from build123d import *

# Parameters (mm, degrees)
BOSS_EXTRUDE1_DEPTH   = 30
SKETCH2_R             = 3
CUT_EXTRUDE1_DEPTH    = 30
SKETCH3_R             = 9.5
CUT_EXTRUDE2_DEPTH    = 6
SKETCH4_R             = 9.5
CUT_EXTRUDE3_DEPTH    = 6
CUT_EXTRUDE4_REACH    = 26
SKETCH5_R             = 5
SKETCH6_W             = 110
SKETCH6_H             = 20
CUT_EXTRUDE5_DEPTH    = 12
SKETCH7_W             = 110
SKETCH7_H             = 20
CUT_EXTRUDE6_DEPTH    = 12
SKETCH8_W             = 12
SKETCH8_H             = 30
BOSS_EXTRUDE2_DEPTH   = 32
CUT_EXTRUDE7_DEPTH    = 35
BOSS_EXTRUDE3_DEPTH   = 50
SKETCH11_R            = 1.5
CUT_EXTRUDE8_DEPTH    = 10
SKETCH13_R            = 1.5
CUT_EXTRUDE9_DEPTH    = 10
SKETCH12_R            = 1.5
CUT_EXTRUDE10_DEPTH   = 10
BODY_MOVE_COPY1_ANGLE = 90


with BuildPart() as part:
    # Sketch1 → Boss-Extrude1 (new body)
    with BuildSketch(Plane(origin=(0, 0, 0), x_dir=(0, 0, -1), z_dir=(1, 0, 0))):
        with BuildLine():
            Line((0, 30), (135, 30))
            ThreePointArc((135, 30), (150, 15), (135, 0))
            Line((135, 0), (0, 0))
            ThreePointArc((0, 0), (-15, 15), (0, 30))
        make_face()
    extrude(amount=BOSS_EXTRUDE1_DEPTH)

    # Sketch2 → Cut-Extrude1 (cut)
    with BuildSketch(Plane(origin=(30, 0, 0), x_dir=(0, 0, -1), z_dir=(1, 0, 0))):
        with Locations((0, 15)):
            Circle(SKETCH2_R)
    extrude(amount=-CUT_EXTRUDE1_DEPTH, mode=Mode.SUBTRACT)

    # Sketch3 → Cut-Extrude2 (cut)
    with BuildSketch(Plane(origin=(30, 0, 0), x_dir=(0, 0, -1), z_dir=(1, 0, 0))):
        with Locations((135, 15)):
            Circle(SKETCH3_R)
    extrude(amount=-CUT_EXTRUDE2_DEPTH, mode=Mode.SUBTRACT)

    # Sketch4 → Cut-Extrude3 (cut)
    with BuildSketch(Plane.ZY):
        with Locations((-135, 15)):
            Circle(SKETCH4_R)
    extrude(amount=-CUT_EXTRUDE3_DEPTH, mode=Mode.SUBTRACT)

    # Sketch5 → Cut-Extrude4 (cut, up to next)
    with BuildSketch(Plane.ZY.offset(-6), mode=Mode.PRIVATE) as cut_extrude4_sk1:
        with Locations((-135, 15)):
            Circle(SKETCH5_R)
    cut_extrude4_tool1 = extrude(cut_extrude4_sk1.sketch, amount=-CUT_EXTRUDE4_REACH, mode=Mode.PRIVATE) & part.part
    add(cut_extrude4_tool1.solids().sort_by_distance((6, 15, -135))[0], mode=Mode.SUBTRACT)

    # Sketch6 → Cut-Extrude5 (cut)
    with BuildSketch(Plane(origin=(30, 0, 0), x_dir=(0, 0, -1), z_dir=(1, 0, 0))):
        with Locations((67.5, 15)):
            Rectangle(SKETCH6_W, SKETCH6_H)
    extrude(amount=-CUT_EXTRUDE5_DEPTH, mode=Mode.SUBTRACT)

    # Sketch7 → Cut-Extrude6 (cut)
    with BuildSketch(Plane.ZY):
        with Locations((-67.5, 15)):
            Rectangle(SKETCH7_W, SKETCH7_H)
    extrude(amount=-CUT_EXTRUDE6_DEPTH, mode=Mode.SUBTRACT)

    # Sketch8 → Boss-Extrude2 (add)
    with BuildSketch(Plane.ZY.offset(-12)):
        with Locations((-97, 15)):
            Rectangle(SKETCH8_W, SKETCH8_H)
        with Locations((-151, 15)):
            Rectangle(SKETCH8_W, SKETCH8_H)
    extrude(amount=BOSS_EXTRUDE2_DEPTH)

    # Sketch9 → Cut-Extrude7 (cut)
    with BuildSketch(Plane(origin=(12, 0, 0), x_dir=(0, 0, -1), z_dir=(1, 0, 0))):
        with BuildLine():
            Line((145, 30), (145, 26.180339887))
            ThreePointArc((145, 26.180339887), (150, 15), (145, 3.819660113))
            Line((145, 3.819660113), (145, 0))
            Line((145, 0), (157, 0))
            Line((157, 0), (157, 30))
            Line((157, 30), (145, 30))
        make_face()
    extrude(amount=-CUT_EXTRUDE7_DEPTH, mode=Mode.SUBTRACT)

    # Sketch10 → Boss-Extrude3 (add)
    with BuildSketch(Plane(origin=(30, 0, 0), x_dir=(0, 0, -1), z_dir=(1, 0, 0))):
        with BuildLine():
            Line((135, 30), (145, 30))
            ThreePointArc((145, 30), (160, 15), (145, 0))
            Line((145, 0), (135, 0))
            ThreePointArc((135, 0), (150, 15), (135, 30))
        make_face()
    extrude(amount=-BOSS_EXTRUDE3_DEPTH)

    # Sketch11 → Cut-Extrude8 (cut)
    with BuildSketch(Plane.ZY.offset(20)):
        with Locations((-149.85, 10.350189987)):
            Circle(SKETCH11_R)
    extrude(amount=-CUT_EXTRUDE8_DEPTH, mode=Mode.SUBTRACT)

    # Sketch13 → Cut-Extrude9 (cut)
    with BuildSketch(Plane.ZY.offset(20)):
        with Locations((-149.85, 20.350189987)):
            Circle(SKETCH13_R)
        with Locations((-99.35, 20.350189987)):
            Circle(SKETCH13_R)
    extrude(amount=-CUT_EXTRUDE9_DEPTH, mode=Mode.SUBTRACT)

    # Sketch12 → Cut-Extrude10 (cut)
    with BuildSketch(Plane.ZY.offset(20)):
        with Locations((-99.35, 10.350189987)):
            Circle(SKETCH12_R)
    extrude(amount=-CUT_EXTRUDE10_DEPTH, mode=Mode.SUBTRACT)


with BuildPart() as part_1:
    # Body-Move/Copy1: moved
    add(part.part.rotate(Axis((5, 0, -72.5), (0, -1, 0)), BODY_MOVE_COPY1_ANGLE))


with BuildPart() as part_2:
    # Body-Move/Copy2: moved
    add(part_1.part.moved(Location((67.5, -15, 47.5))))


solid = part_2.part
The model under review builds one solid part; all positions refer to its coordinate system, in mm. A direction names the side the tool comes from. Give positions to 0.01 mm unless a question says otherwise; leave off trailing zeros. Order: outer loops, then holes, each group sorted by start corner. A loop starts at its lowest first (then second) coordinate and runs counter-clockwise, first axis right, second up. Notation, with made-up numbers: (9, -36.5) -> (53, -36.5) arc R8 cw to (53, -21.5) -> close; hole circle Ø4 at (85, 20.25). An arc over 180 degrees is marked (long way). Write item = value, one per line. Start each with the question number.
(1) Take a section at A-A (z = -45). Write out the cut boundary in (x, y).
(2) For L1, parallel to Y at x = 135, z = -15.5; L2, parallel to X at y = 3.75, z = -22; L3, parallel to Y at x = 99.35, z = -43.5, list the stretches that pass through material, from the lowest coordinate up. Write a range as from..to.
(3) Tool access review of faces 4 (the cylindrical face through (151.35, -4.58, -45.07)), 5 (the cylindrical face through (125.51, 0.42, -2.96)), 6 (the flat face through (27, 10.2, -30)), 7 (the cylindrical face through (130.23, 1.5, -15.13)): name each direction out of +Z, -Z, +X, -X, +Y, -Y from which nothing blocks a thin tool from reaching the whole face with its end or side.
(4) Take a section at C-C (z = -31.5). Write out the cut boundary in (x, y).
(5) Draft analysis for pull direction X (two halves, no side actions). For faces 1 (the cylindrical face through (-15, 0, -15)), 2 (the flat face through (67, 10, -6)), 3 (the flat face through (150, 0, -50)), state which applies: +X half, -X half, draft (parallel to the pull), parting line (faces both ways), or undercut.
(6) Take a section at B-B (y = 0). State how many separate pieces and enclosed holes the cut face has, plus the area to 3 significant figures.
(7) For pin 1 Ø16 at (x, y) = (135, 0) entering from +Z; pin 2 Ø15 at (x, y) = (131, 3) entering from -Z; pin 3 Ø1.5 at (x, y) = (84, -3.5) entering from -Z, all flat-tipped, find the tip position at first contact; note any pin that passes through.
(8) Take a section at D-D (x = 117). Write out the cut boundary in (y, z), plus the area to 3 significant figures.
Returned:
q1.outline = (91, -15) -> (103, -15) -> (103, 15) -> (91, 15) -> close; (135, -15) -> (145, -15) arc R15 ccw to (145, 15) -> (135, 15) arc R15 cw to (145, 11.18) -> (145, -11.18) arc R15 cw to start; hole circle Ø3 at (99.35, -4.65); hole circle Ø3 at (99.35, 5.35); hole circle Ø3 at (149.85, -4.65); hole circle Ø3 at (149.85, 5.35)
q2.L1 = -15..-5, 5..15
q2.L2 = -14.52..12.5, 91..103, 122.5..131.69, 138.31..159.52
q2.L3 = -15..-6.15, -3.15..3.85, 6.85..15
q3.face_4 = -Z
q3.face_5 = +Z
q3.face_6 = -Z, -X, +Y, -Y
q3.face_7 = +Z, -Z
q4.outline = (91, -15) -> (103, -15) -> (103, 15) -> (91, 15) -> close; (135, -15) -> (145, -15) arc R15 ccw to (145, 15) -> (135, 15) arc R15 cw to (145, 11.18) -> (145, -11.18) arc R15 cw to start
q5.face_1 = -X half
q5.face_2 = undercut
q5.face_3 = draft
q6.separate_pieces = 3
q6.enclosed_holes = 0
q6.area = 2,710 mm²
q7.pin_1 = -6
q7.pin_2 = -30
q7.pin_3 = -18
q8.outline = (-15, -30) -> (-10, -30) -> (-10, -18) -> (10, -18) -> (10, -30) -> (15, -30) -> (15, 0) -> (10, 0) -> (10, -12) -> (-10, -12) -> (-10, 0) -> (-15, 0) -> close
q8.area = 420 mm²
